from build123d import *

# Parameters (mm, degrees)
F0_W         = 30
F0_H         = 25
F1_DEPTH     = 17
F3_DEPTH     = 50
F4_D         = 5
F5_R         = 2.5
F6_DEPTH     = 6
F7_R         = 5
F8_T1_DEPTH  = 40
F8_T3_DEPTH  = 20
F8_T6_ANGLE  = 90
F8_T8_ANGLE  = 90
F8_T10_ANGLE = 90
F8_T12_ANGLE = 90


# Not quite as in the source:
# - a fillet or chamfer that OpenCascade refuses, or shapes differently, is made with other operations: its cross-section is extruded or revolved along the edge and cut away or added


with BuildPart() as f1:
    # F0 (on Top) → F1 (new body)
    with BuildSketch(Plane.XY):
        with Locations((0, 12.5)):
            Rectangle(F0_W, F0_H)
        with Locations((0, -12.5)):
            Rectangle(F0_W, F0_H)
    extrude(amount=F1_DEPTH)

    # F2 (on face) → F3 (cut)
    with BuildSketch(Plane.YZ.offset(15)):
        with BuildLine():
            Line((-11.5, 0), (11.5, 0))
            ThreePointArc((11.5, 0), (0, 11.5), (-11.5, 0))
        make_face()
        with BuildLine():
            ThreePointArc((-11.5, 0), (0, -11.5), (11.5, 0))
            Line((11.5, 0), (-11.5, 0))
        make_face()
    extrude(amount=-F3_DEPTH, mode=Mode.SUBTRACT)

    # F4 (through all)
    with Locations(Plane(origin=(0, 0, 0), x_dir=(1, 0, 0), z_dir=(0, 0, -1))):
        with Locations((0, -19), (0, 19)):
            Hole(F4_D / 2)

    # F5 (on face) → F6 (cut)
    with BuildSketch(Plane.XY.offset(17)):
        Polygon((4, -21.3094010768), (4, -16.6905989232), (0, -14.3811978465), (-4, -16.6905989232), (-4, -21.3094010768), (0, -23.6188021535), align=None)
        with Locations((0, -19)):
            Circle(F5_R, mode=Mode.SUBTRACT)
        Polygon((4, 16.6905989232), (4, 21.3094010768), (0, 23.6188021535), (-4, 21.3094010768), (-4, 16.6905989232), (0, 14.3811978465), align=None)
        with Locations((0, 19)):
            Circle(F5_R, mode=Mode.SUBTRACT)
    extrude(amount=-F6_DEPTH, mode=Mode.SUBTRACT)

    # F7
    f7_edges = [f1.edges().sort_by_distance(p)[0] for p in [
        (-15, 25, 8.5),
        (15, 25, 8.5),
        (-15, -25, 8.5),
        (15, -25, 8.5),
    ]]
    fillet(f7_edges, radius=F7_R)

    # F8: fillet of radius 5 on 1 edges, made by hand

    # F8_s2 → F8_t1 (cut)
    with BuildSketch(Plane.XZ.offset(-20)):
        with BuildLine():
            ThreePointArc((-15, 12), (-13.5355339059, 15.5355339059), (-10, 17))
            Line((-10, 17), (-15, 17))
            Line((-15, 17), (-15, 12))
        make_face()
        with BuildLine():
            ThreePointArc((10, 17), (13.5355339059, 15.5355339059), (15, 12))
            Line((15, 12), (15, 17))
            Line((15, 17), (10, 17))
        make_face()
    extrude(amount=F8_T1_DEPTH, mode=Mode.SUBTRACT)

    # F8_s4 → F8_t3 (cut)
    with BuildSketch(Plane.YZ.offset(-10)):
        with BuildLine():
            ThreePointArc((-20, 17), (-23.5355339059, 15.5355339059), (-25, 12))
            Line((-25, 12), (-25, 17))
            Line((-25, 17), (-20, 17))
        make_face()
        with BuildLine():
            ThreePointArc((20, 17), (23.5355339059, 15.5355339059), (25, 12))
            Line((25, 12), (25, 17))
            Line((25, 17), (20, 17))
        make_face()
    extrude(amount=F8_T3_DEPTH, mode=Mode.SUBTRACT)

    # F8_s5 → F8_t6 (revolve, cut)
    with BuildSketch(Plane.XZ.offset(-20)):
        with BuildLine():
            ThreePointArc((-15, 12), (-13.5355339059, 15.5355339059), (-10, 17))
            Line((-10, 17), (-15, 17))
            Line((-15, 17), (-15, 12))
        make_face()
    revolve(axis=Axis((-10, 20, 17), (0, 0, -1)), revolution_arc=F8_T6_ANGLE, mode=Mode.SUBTRACT)

    # F8_s7 → F8_t8 (revolve, cut)
    with BuildSketch(Plane.XZ.offset(20)):
        with BuildLine():
            ThreePointArc((-10, 17), (-13.5355339059, 15.5355339059), (-15, 12))
            Line((-15, 12), (-15, 17))
            Line((-15, 17), (-10, 17))
        make_face()
    revolve(axis=Axis((-10, -20, 17), (0, 0, 1)), revolution_arc=F8_T8_ANGLE, mode=Mode.SUBTRACT)

    # F8_s9 → F8_t10 (revolve, cut)
    with BuildSketch(Plane.YZ.offset(10)):
        with BuildLine():
            ThreePointArc((-20, 17), (-23.5355339059, 15.5355339059), (-25, 12))
            Line((-25, 12), (-25, 17))
            Line((-25, 17), (-20, 17))
        make_face()
    revolve(axis=Axis((10, -20, 17), (0, 0, 1)), revolution_arc=F8_T10_ANGLE, mode=Mode.SUBTRACT)

    # F8_s11 → F8_t12 (revolve, cut)
    with BuildSketch(Plane.YZ.offset(10)):
        with BuildLine():
            ThreePointArc((20, 17), (23.5355339059, 15.5355339059), (25, 12))
            Line((25, 12), (25, 17))
            Line((25, 17), (20, 17))
        make_face()
    revolve(axis=Axis((10, 20, 17), (0, 0, -1)), revolution_arc=F8_T12_ANGLE, mode=Mode.SUBTRACT)


solid = f1.part
The listing builds one solid part. Answer for the finished solid, in the listing's coordinates (mm). A direction names the side the tool comes from. Round coordinates to 2 decimals unless told otherwise and drop trailing zeros. Order: outer loops, then holes, each group sorted by start corner. A loop starts at its lowest first (then second) coordinate and runs counter-clockwise, first axis right, second up. Notation, with made-up numbers: (-20.5, 84.25) -> (23.5, 84.25) arc R11 ccw to (23.5, 97.25) -> close; hole circle Ø8 at (-31, 36.5). An arc over 180 degrees is marked (long way). Write each question's results on one line, items separated by ' | '. Start each with the question number.
Q1. Find section C-C (x = -1). Determine the outline of the cut face in (y, z), then the cut area to 3 significant figures.
Q2. Each of these flat-tipped pins is pushed along its axis until it touches: pin 1 (3 mm diameter, centred on x = 0, y = -19, fed in from +Z) (1 decimal); pin 2 (1 mm diameter, centred on x = 10.5, z = 13, fed in from -Y); pin 3 (2.5 mm diameter, centred on x = -1, y = -20, fed in from +Z); pin 4 (6.5 mm diameter, centred on x = -0.5, y = 20.5, fed in from +Z). Where does it stop, or does it pass through?
Q3. The mould has two halves that part along Y. Classify faces 3 (the flat face through (0, -25, 6)), 4 (the flat face through (0, -15, 0)), 5 (the flat face through (4, -19, 14)): pulls with the +Y half, pulls with the -Y half, needs draft (parallel to the pull), parting line crosses it, or undercut.
Q4. Find section B-B (z = 3.75). Determine the outline of the cut face in (x, y).
Q5. Straight lines are drawn through the part: probe 1 along X at (y, z) = (19, 5); probe 2 along Y at (x, z) = (0, 5); probe 3 along Y at (x, z) = (-1.25, 10.5). For each, find the intervals that lie inside material, in ascending order. Write a range as from..to.
Q6. Which of the six approach directions +Z, -Z, +X, -X, +Y, -Y give full straight-line access (tool end or side, diameter ignored) to faces 1 (the flat face through (-15, 5, 11)), 2 (the flat face through (-1.97, -15.52, 14.04))?
Q7. Find section A-A (y = -19). Determine the outline of the cut face in (x, z).
Q8. Find section D-D (y = 0). Determine the outline of the cut face in (x, z), then the cut area to 3 significant figures.
Worked answers:
1) outline: (-25, 0) -> (-21.29, 0) -> (-21.29, 11) -> (-23.04, 11) -> (-23.04, 15.97) arc R5 ccw to (-25, 12) -> close; (-16.71, 0) -> (-11.5, 0) arc R11.5 cw to (11.5, 0) -> (16.71, 0) -> (16.71, 11) -> (14.96, 11) -> (14.96, 17) -> (-14.96, 17) -> (-14.96, 11) -> (-16.71, 11) -> close; (21.29, 0) -> (25, 0) -> (25, 12) arc R5 ccw to (23.04, 15.97) -> (23.04, 11) -> (21.29, 11) -> close | area: 436 mm2
2) pin 1: passes through | pin 2: stops at y = -24.96 | pin 3: stops at z = 11 | pin 4: stops at z = 16.75
3) face 3: pulls with the -Y half | face 4: needs draft | face 5: undercut
4) outline: (-15, -20) arc R5 ccw to (-10, -25) -> (10, -25) arc R5 ccw to (15, -20) -> (15, -10.87) -> (-15, -10.87) -> close; (-15, 10.87) -> (15, 10.87) -> (15, 20) arc R5 ccw to (10, 25) -> (-10, 25) arc R5 ccw to (-15, 20) -> close; hole circle Ø5 at (0, -19); hole circle Ø5 at (0, 19)
5) probe 1: x = -15..-2.5, 2.5..15 | probe 2: y = -25..-21.5, -16.5..-10.36, 10.36..16.5, 21.5..25 | probe 3: y = -25..-21.17, -16.83..-4.69, 4.69..16.83, 21.17..25
6) face 1: +Z, -Z, -X, +Y, -Y | face 2: +Z
7) outline: (-15, 0) -> (-2.5, 0) -> (-2.5, 11) -> (-4, 11) -> (-4, 17) -> (-10, 17) arc R5 ccw to (-15, 12) -> close; (2.5, 0) -> (15, 0) -> (15, 12) arc R5 ccw to (10, 17) -> (4, 17) -> (4, 11) -> (2.5, 11) -> close
8) outline: (-15, 11.5) -> (15, 11.5) -> (15, 12) arc R5 ccw to (10, 17) -> (-10, 17) arc R5 ccw to (-15, 12) -> close | area: 154 mm2
